Geometry check sheet. Reference: the model listing, model coordinates, mm. Coordinates: 2 decimals unless noted, no trailing zeros. Write each loop counter-clockwise with the first axis right and the second up, starting at its lowest first coordinate (ties: lowest second). Pieces come first, ordered by that corner, then holes. Notation, with made-up numbers: (-39.5, 41) -> (5.5, 41) arc R33 ccw to (5.5, 77) -> close; hole circle Ø10 at (52.5, 9.25). An arc over 180 degrees is marked (long way). One line per question, with ' | ' between items.
from build123d import *

# Parameters (mm, degrees)
SKETCH1_W           = 69.596
SKETCH1_H           = 20.4724
BOSS_EXTRUDE1_DEPTH = 3.175


with BuildPart() as part:
    # Sketch1 → Boss-Extrude1 (new body)
    with BuildSketch(Plane(origin=(0, 0, 0), x_dir=(1, 0, 0), z_dir=(0, 1, 0))):
        Polygon((272.33503015, 4.835931583), (136.08943015, -52.902160647), (110.68943015, -52.902160647), (110.68943015, -56.077160647), (85.28943015, -56.077160647), (85.28943015, -52.902160647), (-84.25556985, -52.902160647), (-84.25556985, -56.077160647), (-109.65556985, -56.077160647), (-109.65556985, -52.902160647), (-135.05556985, -52.902160647), (-135.05556985, -27.502160647), (-138.23056985, -27.502160647), (-138.23056985, -2.102160647), (-135.05556985, -2.102160647), (-135.05556985, 77.272839353), (-138.23056985, 77.272839353), (-138.23056985, 102.672839353), (-135.05556985, 102.672839353), (-135.05556985, 128.072839353), (-84.25556985, 128.072839353), (-84.25556985, 131.247839353), (-33.45556985, 131.247839353), (-33.45556985, 128.072839353), (136.08943015, 128.072839353), (170.73503015, 128.072839353), (170.73503015, 131.247839353), (221.53503015, 131.247839353), (221.53503015, 128.072839353), (272.33503015, 128.072839353), align=None)
        Polygon((201.03723015, 54.782902056), (250.077682757, 11.185931583), (151.996777543, 11.185931583), align=None, mode=Mode.SUBTRACT)
        Polygon((-56.511497321, -7.029760647), (-40.05956985, -7.029760647), (-40.05956985, -17.265960647), (-43.23456985, -17.265960647), (-43.23456985, -29.965960647), (-40.05956985, -29.965960647), (-40.05956985, -40.202160647), (117.648185377, -40.202160647), (3.69193015, 30.123488044), align=None, mode=Mode.SUBTRACT)
        Polygon((210.594577543, 63.279385468), (259.63503015, 19.682414995), (259.63503015, 106.87635594), align=None, mode=Mode.SUBTRACT)
        Polygon((142.43943015, -1.514068417), (142.43943015, -36.417831993), (224.802459945, -1.514068417), align=None, mode=Mode.SUBTRACT)
        Polygon((151.996777543, 115.372839353), (250.077682757, 115.372839353), (201.03723015, 71.77586888), align=None, mode=Mode.SUBTRACT)
        Polygon((142.43943015, 106.87635594), (142.43943015, 19.682414995), (191.479882757, 63.279385468), align=None, mode=Mode.SUBTRACT)
        Polygon((-110.264325076, 115.372839353), (117.648185377, 115.372839353), (3.69193015, 45.047190661), align=None, mode=Mode.SUBTRACT)
        Polygon((-122.35556985, 107.910988044), (-122.35556985, -7.029760647), (-122.35556985, -10.204760647), (-80.693986868, -10.204760647), (-80.693986868, -7.029760647), (-8.399314623, 37.585339353), align=None, mode=Mode.SUBTRACT)
        Polygon((129.73943015, 107.910988044), (129.73943015, -32.740309339), (15.783174924, 37.585339353), align=None, mode=Mode.SUBTRACT)
        with Locations((-87.55756985, -29.965960647)):
            Rectangle(SKETCH1_W, SKETCH1_H, mode=Mode.SUBTRACT)
    extrude(amount=BOSS_EXTRUDE1_DEPTH)


solid = part.part
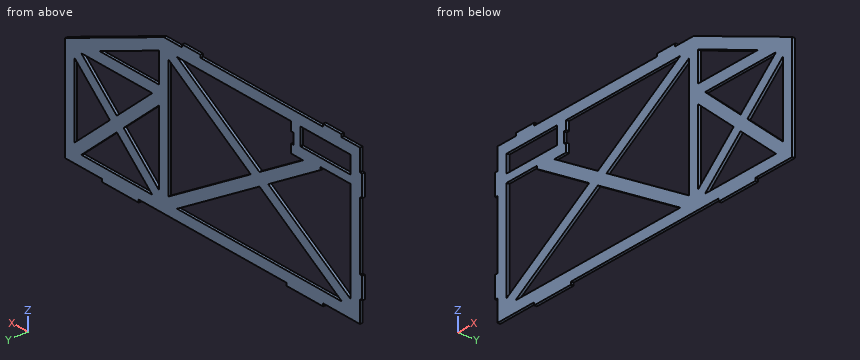
1. Cross-section at A-A on x = 147.5. Record the boundary of the cut face in (y, z) (1 decimal), and give its area (3 significant figures).
Worked answers:
outline: (0, -128.1) -> (3.2, -128.1) -> (3.2, -102.4) -> (0, -102.4) -> close; (0, -24.2) -> (3.2, -24.2) -> (3.2, 1.5) -> (0, 1.5) -> close; (0, 34.3) -> (3.2, 34.3) -> (3.2, 48.1) -> (0, 48.1) -> close | area: 207 mm²
2. Cross-section at C-C on y = 2.45. Give the number of separate pieces and of enclosed holes in the cut face, and give its area (3 significant figures).
Worked answers:
separate pieces: 1 | enclosed holes: 10 | area: 28,800 mm²
3. Go/stop test with flat-tipped pins: P1, Ø1, axis at x = -97.5, y = 1.5, coming from the -Z side; P2, Ø1, axis at y = 2, z = 16.5, coming from the +X side; P3, Ø1, axis at x = -41.5, y = 1.5, coming from the +Z side. Record where each tip stops, or that it passes through.
Worked answers:
P1: z = -128.07 | P2: x = 223.17 | P3: z = 52.9
4. Cross-section at B-B on z = -15.5. Record the boundary of the cut face in (x, y) (1 decimal), and give its area (3 significant figures).
Worked answers:
outline: (-135.1, 0) -> (-122.4, 0) -> (-122.4, 3.2) -> (-135.1, 3.2) -> close; (-44.2, 0) -> (-20, 0) -> (-20, 3.2) -> (-44.2, 3.2) -> close; (27.4, 0) -> (51.6, 0) -> (51.6, 3.2) -> (27.4, 3.2) -> close; (129.7, 0) -> (156.8, 0) -> (156.8, 3.2) -> (129.7, 3.2) -> close; (245.2, 0) -> (272.3, 0) -> (272.3, 3.2) -> (245.2, 3.2) -> close | area: 366 mm²
5. Material ranges on line 1 (X direction, y = 0.7, z = -59.5); line 2 (Z direction, x = -9.5, y = 1.8); line 3 (X direction, y = 1.8, z = 20), recorded low to high. Write a range as from..to.
Worked answers:
line 1: -135.06..-122.36, -43.91..-19.73, 27.11..51.29, 129.74..142.44, 187.23..214.85, 259.64..272.34 | line 2: -128.07..-115.37, -53.19..-38.26, -36.91..-21.98, 40.2..52.9 | line 3: -138.23..-122.36, -52.76..-43.23, 84.91..109.09, 129.74..142.44, 181.18..213.73
